```python
from build123d import *

# Parameters (mm, degrees)
CUT_EXTRUDE1_START = 1.397
CUT_EXTRUDE1_DEPTH = 10.7188
CIRPATTERN1_COUNT  = 24
SKETCH4_R          = 1.5875
CUT_EXTRUDE2_DEPTH = 34.439119294
CUT_EXTRUDE3_DEPTH = 1.190625
CIRPATTERN2_COUNT  = 2
CIRPATTERN2_ANGLE  = 90
SKETCH7_R          = 13.5001
CUT_EXTRUDE4_DEPTH = 7.9248
CUT_EXTRUDE5_DEPTH = 35.629218341


with BuildPart() as part:
    # Sketch2 → Revolve1 (revolve)
    with BuildSketch(Plane(origin=(0, 0, 0), x_dir=(0, 0, -1), z_dir=(1, 0, 0)), mode=Mode.PRIVATE) as revolve1_sk:
        with BuildLine():
            Line((-11.1125, 3.175), (11.1125, 3.175))
            Line((11.1125, 3.175), (11.1125, 22.3012))
            Line((11.1125, 22.3012), (10.21715, 22.3012))
            ThreePointArc((10.21715, 22.3012), (9.559608575, 21.573014266), (9.3218, 20.621141234))
            Line((9.3218, 20.621141234), (9.3218, 18.941082468))
            Line((9.3218, 18.941082468), (-1.397, 18.941082468))
            Line((-1.397, 18.941082468), (-1.397, 20.621141234))
            ThreePointArc((-1.397, 20.621141234), (-1.634808575, 21.573014266), (-2.29235, 22.3012))
            Line((-2.29235, 22.3012), (-3.1877, 22.3012))
            Line((-3.1877, 22.3012), (-3.1877, 13.5001))
            Line((-3.1877, 13.5001), (-11.1125, 13.5001))
            Line((-11.1125, 13.5001), (-11.1125, 3.175))
        make_face()
    revolve(revolve1_sk.sketch.rotate(Axis((0, 0, 11.1125), (0, 0, -1)), 90), axis=Axis((0, 0, 11.1125), (0, 0, -1)))

    # Sketch3 → Cut-Extrude1 (cut)
    with BuildSketch(Plane.XY.offset(CUT_EXTRUDE1_START)):
        with BuildLine():
            Line((-0.690489274, 17.6276), (0.690489274, 17.6276))
            Line((0.690489274, 17.6276), (1.2827, 18.8976))
            ThreePointArc((1.2827, 18.8976), (0, 18.941082468), (-1.2827, 18.8976))
            Line((-1.2827, 18.8976), (-0.690489274, 17.6276))
        make_face()
    cut_extrude1 = extrude(amount=-CUT_EXTRUDE1_DEPTH, mode=Mode.SUBTRACT)

    # CirPattern1: Cut-Extrude1 ×24 about axis
    cirpattern1_axis = Axis((0, 0, 0), (0, 0, 1))
    for i in range(1, CIRPATTERN1_COUNT):
        add(cut_extrude1.rotate(cirpattern1_axis, i * 360 / CIRPATTERN1_COUNT), mode=Mode.SUBTRACT)

    # Sketch4 → Cut-Extrude2 (cut, through all)
    with BuildSketch(Plane(origin=(0, 0, 0), x_dir=(1, 0, 0), z_dir=(0, 1, 0))):
        with Locations(Location((0, -7.1501, 0), (0, 0, 90))):
            Circle(SKETCH4_R)
    cut_extrude2 = extrude(amount=CUT_EXTRUDE2_DEPTH, mode=Mode.SUBTRACT)

    # Sketch5 → Revolve2 (revolve)
    with BuildSketch(Plane.XY.offset(7.1501), mode=Mode.PRIVATE) as revolve2_sk:
        Polygon((1.0795, 13.406436654), (1.5875, 12.898436654), (1.5875, 3.81), (0.9525, 3.175), (0, 3.175), (0, 13.406436654), align=None)
    revolve2 = revolve(revolve2_sk.sketch.rotate(Axis((0, 0, 7.1501), (0, 1, 0)), 90), axis=Axis((0, 0, 7.1501), (0, 1, 0)))

    # Sketch6 → Cut-Extrude3 (cut)
    with BuildSketch(Plane(origin=(0, 13.406436654, 0), x_dir=(1, 0, 0), z_dir=(0, 1, 0))):
        Polygon((0, -6.233556448), (-0.79375, -6.691828224), (-0.79375, -7.608371776), (0, -8.066643552), (0.79375, -7.608371776), (0.79375, -6.691828224), align=None)
    cut_extrude3 = extrude(amount=-CUT_EXTRUDE3_DEPTH, mode=Mode.SUBTRACT)

    # CirPattern2: Cut-Extrude2, Revolve2, Cut-Extrude3 ×2 about axis
    cirpattern2_axis = Axis((0, 0, 0), (0, 0, -1))
    add([cut_extrude2.rotate(cirpattern2_axis, i * CIRPATTERN2_ANGLE / (CIRPATTERN2_COUNT - 1)) for i in range(1, CIRPATTERN2_COUNT)], mode=Mode.SUBTRACT)
    add([revolve2.rotate(cirpattern2_axis, i * CIRPATTERN2_ANGLE / (CIRPATTERN2_COUNT - 1)) for i in range(1, CIRPATTERN2_COUNT)])
    add([cut_extrude3.rotate(cirpattern2_axis, i * CIRPATTERN2_ANGLE / (CIRPATTERN2_COUNT - 1)) for i in range(1, CIRPATTERN2_COUNT)], mode=Mode.SUBTRACT)

    # Sketch7 → Cut-Extrude4 (cut)
    with BuildSketch(Plane.XY.offset(11.1125)):
        Circle(SKETCH7_R)
    extrude(amount=-CUT_EXTRUDE4_DEPTH, mode=Mode.SUBTRACT)

    # Sketch8 → Cut-Extrude5 (cut, through all)
    with BuildSketch(Plane.XY.offset(3.1877)):
        Polygon((3.886144662, 0), (1.943072331, 3.3655), (-1.943072331, 3.3655), (-3.886144662, 0), (-1.943072331, -3.3655), (1.943072331, -3.3655), align=None)
    extrude(amount=-CUT_EXTRUDE5_DEPTH, mode=Mode.SUBTRACT)


solid = part.part
```
Check sheet for the modelled part. Datum: model origin and axes. Units: mm. A direction names the side the tool comes from. Give positions to 0.01 mm unless a question says otherwise; leave off trailing zeros. Order: outer loops, then holes, each group sorted by start corner. A loop starts at its lowest first (then second) coordinate and runs counter-clockwise, first axis right, second up. Notation, with made-up numbers: M 39,50 L 82,50 A24 cw 82,69 Z; hole C -29,-19 d9. An arc over 180 degrees is marked long. Answer in a Markdown table with one row per item. Add a question column.
Q1. Gauge pin test, flat ends, axial feed: pin 1 Ø1.5 at (x, z) = (4.5, 1.5) entering from +Y; pin 2 Ø1.5 at (x, z) = (-14.5, 1) entering from +Y; pin 3 Ø3 at (x, z) = (-9, -1.5) entering from -Y. Record the tip position at first contact, or that the pin passes through.
Q2. Release check for a two-part mould opening along X. For faces 5 (the flat face through (17.392, 5.686, -3.887)), 6 (the cylindrical face through (-7.264, 17.493, -3.887)), 7 (the flat face through (0.98, 18.25, -3.89)), 8 (the flat face through (-2.93, -1.66, -3.86)) record: released by +X, released by -X, zero draft, split by the parting line, or undercut.
Q3. Sectioned sample at A-A, the plane x = 0. Record the boundary of the cut face in (y, z), and give its area (3 significant figures).
Q4. Thickness scan on L1, parallel to Z at x = 10, y = 17.5; L2, parallel to X at y = 2, z = -9.5; L3, parallel to Y at x = -1, z = -7.75. Record the ranges inside material, lowest first.
Q5. Access from +Z, -Z, +X, -X, +Y, -Y to the whole of each face (thin tool, end or side, straight path). Record for faces 1 (the flat face through (-2.9, 1.71, -3.86)), 2 (the cylindrical face through (-2.46, -18.78, -3.89)), 3 (the flat face through (-17.886, -3.775, -3.887)), 4 (the flat face through (12.22, 13.62, -3.89)).
Verdict:
| question | item | result |
|---|---|---|
| 1 | pin 1 | y = 21.83 |
| 1 | pin 2 | y = 16.36 |
| 1 | pin 3 | y = -17.39 |
| 2 | face 5 | released by +X |
| 2 | face 6 | released by -X |
| 2 | face 7 | undercut |
| 2 | face 8 | undercut |
| 3 | outline | M -22.3,-11.11 L -3.37,-11.11 L -3.37,3.19 L -22.3,3.19 L -22.3,2.29 A2.02 ccw -20.62,1.4 L -17.63,1.4 L -17.63,-9.32 L -20.62,-9.32 A2.02 ccw -22.3,-10.22 Z; M 3.37,-11.11 L 22.3,-11.11 L 22.3,-10.22 A2.02 ccw 20.62,-9.32 L 17.63,-9.32 L 17.63,1.4 L 20.62,1.4 A2.02 ccw 22.3,2.29 L 22.3,3.19 L 3.37,3.19 Z |
| 3 | area | 440 mm² |
| 4 | L1 | -11.11 to -9.32, 1.4 to 3.19 |
| 4 | L2 | -21.36 to -2.73, 2.73 to 21.36 |
| 4 | L3 | -18.29 to -3.37, 3.37 to 18.29 |
| 5 | face 1 | +Z, -Z |
| 5 | face 2 | -X, -Y |
| 5 | face 3 | -X |
| 5 | face 4 | +X |
